from build123d import *

# Parameters (mm, degrees)
EXTRUDE_1_DEPTH             = 12
SKETCH_2_W                  = 18
SKETCH_2_H                  = 50
EXTRUDE_3_REACH             = 84.006
SKETCH_3_R                  = 12
EXTRUDE_3_DIRECTION_2_REACH = 84.006
EXTRUDE_4_DEPTH             = 4
RIB_1_REACH                 = 84.006
SKETCH_5_WALL_W             = 174.012194852
SKETCH_5_WALL_H             = 8
HOLE_WIZARD_10_0_10_1_D     = 10
PATTERN_LINEAR_2_COUNT      = 2
PATTERN_LINEAR_2_PITCH      = 80
PATTERN_LINEAR_2_COUNT_DIR2 = 2
PATTERN_LINEAR_2_PITCH_DIR2 = 30
CUT_EXTRUDE_1_DEPTH         = 84.312664198
HOLE_WIZARD_25_0_25_1_D     = 25
HOLE_WIZARD_12_0_12_1_D     = 12


with BuildPart() as part:
    # 草图1 → 凸台-拉伸1 (new body)
    with BuildSketch(Plane(origin=(0, 0, 0), x_dir=(1, 0, 0), z_dir=(0, 1, 0))):
        with BuildLine():
            Line((-50, -25), (30, -25))
            ThreePointArc((30, -25), (37.071067812, -22.071067812), (40, -15))
            Line((40, -15), (40, 15))
            ThreePointArc((40, 15), (37.071067812, 22.071067812), (30, 25))
            Line((30, 25), (-50, 25))
            ThreePointArc((-50, 25), (-57.071067812, 22.071067812), (-60, 15))
            Line((-60, 15), (-60, -15))
            ThreePointArc((-60, -15), (-57.071067812, -22.071067812), (-50, -25))
        make_face()
    extrude(amount=EXTRUDE_1_DEPTH)

    # 草图2 → 旋转1 (revolve)
    with BuildSketch(Plane.XY, mode=Mode.PRIVATE) as revolve_1_sk:
        with Locations((9, 25)):
            Rectangle(SKETCH_2_W, SKETCH_2_H)
    revolve(revolve_1_sk.sketch.rotate(Axis((0, 42.98545342, 0), (0, -1, 0)), 90), axis=Axis((0, 42.98545342, 0), (0, -1, 0)))

    # 凸台-拉伸3: up to this face of the body (flat: up to its plane)
    extrude_3_end = Plane(part.part.faces().sort_by_distance((-10, 6, 25))[0])
    # 草图3 → 凸台-拉伸3 (add, up to the picked face)
    with BuildSketch(Plane.XY, mode=Mode.PRIVATE) as extrude_3_sk1:
        with Locations(Location((0, 32, 0), (0, 0, 180))):
            Circle(SKETCH_3_R)
    extrude_3_tool1 = split(extrude(extrude_3_sk1.sketch, amount=EXTRUDE_3_REACH, mode=Mode.PRIVATE), bisect_by=extrude_3_end, keep=Keep.BOTH, mode=Mode.PRIVATE)
    add(extrude_3_tool1.solids().sort_by(Axis((0, 32, 0), (0, 0, 1)))[0])

    # 凸台-拉伸3 direction 2: up to this face of the body (flat: up to its plane)
    extrude_3_direction_2_end = Plane(part.part.faces().sort_by_distance((-10, 6, -25))[0])
    # 草图3 → 凸台-拉伸3 direction 2 (add, up to the picked face)
    with BuildSketch(Plane.XY, mode=Mode.PRIVATE) as extrude_3_direction_2_sk1:
        with Locations(Location((0, 32, 0), (0, 0, 180))):
            Circle(SKETCH_3_R)
    extrude_3_direction_2_tool1 = split(extrude(extrude_3_direction_2_sk1.sketch, amount=-EXTRUDE_3_DIRECTION_2_REACH, mode=Mode.PRIVATE), bisect_by=extrude_3_direction_2_end, keep=Keep.BOTH, mode=Mode.PRIVATE)
    add(extrude_3_direction_2_tool1.solids().sort_by(Axis((0, 32, 0), (0, 0, -1)))[0])

    # 草图4 → 凸台-拉伸4 (add, symmetric)
    with BuildSketch(Plane.XY):
        with BuildLine():
            Line((-40, 34), (0, 34))
            Line((0, 34), (0, 12))
            Line((0, 12), (-50, 12))
            Line((-50, 12), (-50, 24))
            ThreePointArc((-50, 24), (-47.071067812, 31.071067812), (-40, 34))
        make_face()
    extrude(amount=EXTRUDE_4_DEPTH, both=True)

    # 草图5 wall → 筋1 (add, up to next)
    with BuildSketch(Plane(origin=(0, 16, 25), x_dir=(0, -1, 0), z_dir=(0, 0, -1)), mode=Mode.PRIVATE) as rib_1_sk1:
        Rectangle(SKETCH_5_WALL_W, SKETCH_5_WALL_H)
    rib_1_tool1 = extrude(rib_1_sk1.sketch, amount=RIB_1_REACH, mode=Mode.PRIVATE) - part.part
    rib_1 = rib_1_tool1.solids().sort_by_distance((0, 16, 25))[0]
    add(rib_1)

    # 镜向1: 筋1 across plane
    add(rib_1.mirror(Plane.XY))

    # Ø10.0 (10) 直径孔1 (through all)
    with Locations(Plane(origin=(0, 12, 0), x_dir=(1, 0, 0), z_dir=(0, 1, 0))):
        with Locations((-50, -15)):
            hole_wizard_10_0_10_1 = Hole(HOLE_WIZARD_10_0_10_1_D / 2)

    # 阵列(线性)2: Hole Wizard 10.0 _10_ _1 2 × 2
    with Locations(*[(i * PATTERN_LINEAR_2_PITCH, 0, -j * PATTERN_LINEAR_2_PITCH_DIR2) for i in range(PATTERN_LINEAR_2_COUNT) for j in range(PATTERN_LINEAR_2_COUNT_DIR2) if (i, j) != (0, 0)]):
        add(hole_wizard_10_0_10_1, mode=Mode.SUBTRACT)

    # 草图8 → 切除-拉伸1 (cut, through all)
    with BuildSketch(Plane.XY.offset(4)):
        with BuildLine():
            Line((-39, 18), (-29, 18))
            ThreePointArc((-29, 18), (-24, 23), (-29, 28))
            Line((-29, 28), (-39, 28))
            ThreePointArc((-39, 28), (-44, 23), (-39, 18))
        make_face()
    extrude(amount=-CUT_EXTRUDE_1_DEPTH, mode=Mode.SUBTRACT)

    # Ø25.0 (25) 直径孔1 (through all)
    with Locations(Plane(origin=(0, 50, 0), x_dir=(1, 0, 0), z_dir=(0, 1, 0))):
        with Locations((0, 0)):
            Hole(HOLE_WIZARD_25_0_25_1_D / 2)

    # Ø12.0 (12) 直径孔1 (through all)
    with Locations(Plane.XY.offset(25)):
        with Locations((0, 32)):
            Hole(HOLE_WIZARD_12_0_12_1_D / 2)


solid = part.part
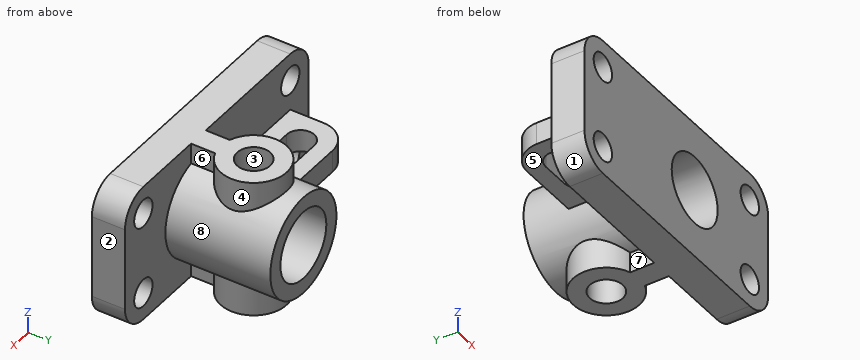
Check sheet for the modelled part. Datum: model origin and axes. Units: mm. Face numbers are marked on the shaded views. A direction names the side the tool comes from. Round coordinates to 2 decimals unless told otherwise and drop trailing zeros. Order: outer loops, then holes, each group sorted by start corner. A loop starts at its lowest first (then second) coordinate and runs counter-clockwise, first axis right, second up.
Q1. Cross-section at B-B, the plane y = 22.5. Enter the section's corners in (x, z).
Filled sheet:
outline: (-50, -4) - (-43.97, -4) - (-43.97, 4) - (-50, 4) - close; (-24.03, -4) - (-17.55, -4) arc R18 ccw to (-7.33, -16.44) - (-7.33, -25) - (7.33, -25) - (7.33, -16.44) arc R18 ccw to (7.33, 16.44) - (7.33, 25) - (-7.33, 25) - (-7.33, 16.44) arc R18 ccw to (-17.55, 4) - (-24.03, 4) - close; hole circle Ø25 at (0, 0)
Q2. Cross-section at C-C, the plane x = 0. Enter the section's corners in (y, z).
Filled sheet:
outline: (0, -25) - (26, -25) - (26, -12.5) - (0, -12.5) - close; (0, 12.5) - (26, 12.5) - (26, 25) - (0, 25) - close; (38, -25) - (44, -25) - (44, -18) - (50, -18) - (50, -12.5) - (38, -12.5) - close; (38, 12.5) - (50, 12.5) - (50, 18) - (44, 18) - (44, 25) - (38, 25) - close
Q3. Depth check by flat-ended pin: P1, Ø5, axis at x = 17.5, z = 14, coming from the +Y side; P2, Ø3, axis at x = -48, z = 13.5, coming from the +Y side; P3, Ø8, axis at y = 18, z = -22.5, coming from the +X side; P4, Ø1.5, axis at y = 31.5, z = 13, coming from the -X side. Enter the tip coordinate at first touch or a pass-through.
Filled sheet:
P1: stops at y = 12
P2: passes through
P3: stops at x = 6.63
P4: stops at x = -13.19
Q4. Cross-section at D-D, the plane y = 32. Enter the section's corners in (x, z), plus the area to 3 significant figures.
Filled sheet:
outline: (-46, -4) - (-17.55, -4) arc R18 ccw to (-12, -13.42) - (-12, -25) - (-6, -25) - (-6, -10.97) arc R12.5 cw to (-6, 10.97) - (-6, 25) - (-12, 25) - (-12, 13.42) arc R18 ccw to (-17.55, 4) - (-46, 4) - close; (6, -25) - (12, -25) - (12, -13.42) arc R18 ccw to (12, 13.42) - (12, 25) - (6, 25) - (6, 10.97) arc R12.5 cw to (6, -10.97) - close
area: 845 mm2
Q5. Cross-section at A-A, the plane z = 0. Enter the section's corners in (x, y), plus the area to 3 significant figures.
Filled sheet:
outline: (-60, 0) - (-12.5, 0) - (-12.5, 50) - (-18, 50) - (-18, 34) - (-40, 34) arc R10 ccw to (-50, 24) - (-50, 12) - (-60, 12) - close; (12.5, 0) - (40, 0) - (40, 12) - (18, 12) - (18, 50) - (12.5, 50) - close; hole (-39, 18) - (-29, 18) arc R5 ccw to (-29, 28) - (-39, 28) arc R5 ccw to start
area: 1,820 mm2
Q6. Scan lines: L1, parallel to Z at x = -50, y = 3; L2, parallel to Y at x = 0, z = 20; L3, parallel to X at y = 3.5, z = -3.5. Record each from-to range of solid material in increasing order.
Filled sheet:
L1: z = -25 to -20, -10 to 10, 20 to 25
L2: y = 0 to 26, 38 to 44
L3: x = -60 to -12, 12 to 40
Q7. Draft check along X on the marked faces 1, 2, 3 and 4. Enter one of: pulls with the +X half, pulls with the -X half, needs draft (parallel to the pull), parting line crosses it, or undercut.
Filled sheet:
face 1: pulls with the -X half
face 2: pulls with the +X half
face 3: undercut
face 4: parting line crosses it
Q8. Set-up check for the marked faces 5, 6, 7 and 8: record each of +Z, -Z, +X, -X, +Y, -Y from which the full face is reachable in a straight line by a thin tool's end or side.
Filled sheet:
face 5: -Z, -X, +Y
face 6: +Z, +X
face 7: -Z, -X
face 8: none
